Geometry: final body of the model. Coordinates: model frame, mm. A direction names the side the tool comes from. Give positions to 0.01 mm unless a question says otherwise; leave off trailing zeros. Order: outer loops, then holes, each group sorted by start corner. A loop starts at its lowest first (then second) coordinate and runs counter-clockwise, first axis right, second up. Notation, with made-up numbers: (-9.75, -31.75) -> (26.25, -31.75) arc R23 cw to (26.25, 0.25) -> close; hole circle Ø6 at (-2.75, 17). An arc over 180 degrees is marked (long way). Write item = value, one per line.
```python
from build123d import *

# Parameters (mm, degrees)
F0_R     = 3.175
F1_DEPTH = 6.35


with BuildPart() as f1:
    # F0 (on Front) → F1 (new body)
    with BuildSketch(Plane.XZ):
        with BuildLine():
            Line((-71.594537, -71.514018), (-71.594537, -84.214018))
            Line((-71.594537, -84.214018), (12.987463, -84.214018))
            Line((12.987463, -84.214018), (12.987463, -71.514018))
            Line((12.987463, -71.514018), (0, -71.514018))
            ThreePointArc((0, -71.514018), (-4.384965, -69.756902), (-6.343192, -65.45798))
            Line((-6.343192, -65.45798), (-11.357634, 42.74481))
            ThreePointArc((-11.357634, 42.74481), (-29.303537, 30.085982), (-47.24944, 42.74481))
            Line((-47.24944, 42.74481), (-52.263882, -65.45798))
            ThreePointArc((-52.263882, -65.45798), (-54.222109, -69.756902), (-58.607074, -71.514018))
            Line((-58.607074, -71.514018), (-71.594537, -71.514018))
        make_face()
        with BuildLine():
            ThreePointArc((-10.253537, 49.135982), (-32.546457, 67.907929), (-47.24944, 42.74481))
            ThreePointArc((-47.24944, 42.74481), (-29.303537, 30.085982), (-11.357634, 42.74481))
            ThreePointArc((-11.357634, 42.74481), (-10.531591, 45.893063), (-10.253537, 49.135982))
        make_face()
        with Locations((-29.303537, 49.135982)):
            Circle(F0_R, mode=Mode.SUBTRACT)
    extrude(amount=-F1_DEPTH)


solid = f1.part
```
1) Mould query, pull axis Z, two halves, no side actions, for faces 4 (the face through (-30, 3, -84.214)), 5 (the face through (-49.72, 3.13, -10.6)), 6 (the face through (-31.644, 3.131, 51.282)), 7 (the face through (12.987, 3, -78)). Classes: +Z half, -Z half, draft (parallel to the pull), parting line (faces both ways), or undercut.
Check sheet entries:
face_4 = -Z half
face_5 = undercut
face_6 = undercut
face_7 = draft
2) Section query C-C (z = -22.5). Output: boundary loops of the cut face in (x, y), plus the area to 3 significant figures.
Check sheet entries:
outline = (-50.27, 0) -> (-8.33, 0) -> (-8.33, 6.35) -> (-50.27, 6.35) -> close
area = 266 mm²
3) Line query: line 1 (Z direction, x = -29.5, y = 1.25); line 2 (X direction, y = 1.5, z = 47); line 3 (Z direction, x = -62.5, y = 5.75). Output: solid intervals per line, ascending. Write a range as from..to.
Check sheet entries:
line_1 = -84.21..45.97, 52.3..68.18
line_2 = -48.23..-31.65, -26.95..-10.37
line_3 = -84.21..-71.51
4) First-contact query: P1, Ø6, axis at x = -7.5, z = -43, coming from the -Y side; P2, Ø1.5, axis at y = 0.5, z = 43.5, coming from the -X side; P3, Ø3, axis at x = 4, y = 4, coming from the +Z side. Flat tips, straight axial feed; report the tip coordinate or a pass-through.
Check sheet entries:
P1 = 0
P2 = -47.72
P3 = -71.51
5) Section query B-B (x = -30). Output: boundary loops of the cut face in (y, z), plus the area to 3 significant figures.
Check sheet entries:
outline = (0, -84.21) -> (6.35, -84.21) -> (6.35, 46.04) -> (0, 46.04) -> close; (0, 52.23) -> (6.35, 52.23) -> (6.35, 68.17) -> (0, 68.17) -> close
area = 928 mm²
6) Section query D-D (z = 35). Output: boundary loops of the cut face in (x, y), plus the area to 3 significant figures.
Check sheet entries:
outline = (-47.61, 0) -> (-11, 0) -> (-11, 6.35) -> (-47.61, 6.35) -> close
area = 232 mm²
7) Reachability of faces 1 (the face through (-65, 3, -71.514)), 2 (the face through (7, 3, -71.514)), 3 (the face through (-10.54, 3.13, 45.85)) from +Z, -Z, +X, -X, +Y, -Y: full face, straight path, thin tool, end or side. Return the list, or none.
Check sheet entries:
face_1 = +Z, -X, +Y, -Y
face_2 = +Z, +X, +Y, -Y
face_3 = +X, +Y, -Y
8) Section query A-A (y = 2). Output: boundary loops of the cut face in (x, z) (3 decimals), plus the area to 3 significant figures.
Check sheet entries:
outline = (-71.595, -84.214) -> (12.987, -84.214) -> (12.987, -71.514) -> (0, -71.514) arc R6.35 cw to (-6.343, -65.458) -> (-11.358, 42.745) arc R19.05 ccw to (-10.254, 49.136) arc R19.05 ccw (long way) to (-47.249, 42.745) -> (-52.264, -65.458) arc R6.35 cw to (-58.607, -71.514) -> (-71.595, -71.514) -> close; hole circle Ø6.35 at (-29.304, 49.136)
area = 6,570 mm²
